Autodesk Inventor part; units mm, degrees
ref_plane "YZ Plane" through (0, 0, 0) normal (1, 0, 0) x (0, 1, 0)
ref_plane "XZ Plane" through (0, 0, 0) normal (0, 1, 0) x (-1, 0, 0)
ref_plane "XY Plane" through (0, 0, 0) normal (0, 0, 1) x (1, 0, 0)
sketch "Boceto1" plane through (0, 0, 0) normal (0, 1, 0) x (-1, 0, 0)
  line L0 (38.5, -14) -> (-38.5, -14)
  line L1 (-38.5, -14) -> (-38.5, 14)
  line L2 (-38.5, 14) -> (38.5, 14)
  line L3 (38.5, 14) -> (38.5, -14)
  circle A0 centre (-29.5, 6) radius 2.5
  circle A1 centre (-29.5, -6) radius 2.5
  point P0 (0, 0)
  point P1 (0, -14)
  point P2 (-38.5, 0)
  dimension "d0" = 5
  dimension "d1" = 9
  dimension "d2" = 77
  dimension "d3" = 28
  dimension "d17" = 8
  dimension "d18" = 5
  dimension "d19" = 12
extrude "Extrusión1" add sketch "Boceto1" along normal blind 9
sketch "Boceto2" plane through (0, 0, 0) normal (0, -1, 0) x (1, 0, 0)
  line L0 (-38.5, 14) -> (38.5, 14)
  line L1 (26.5, 14) -> (32.5, 14)
  line L2 (32.5, 14) -> (32.5, -14)
  line L3 (32.5, -14) -> (26.5, -14)
  line L4 (26.5, -14) -> (26.5, 14)
  line L5 (38.5, -14) -> (-38.5, -14)
  circle A0 centre (29.5, 6) radius 2.5
  circle A1 centre (29.5, -6) radius 2.5
  point P0 (0, 0)
  point P1 (29.5, 14)
  point P2 (26, 6)
  point P3 (31, 6)
  point P4 (26, -6)
  point P5 (31, -6)
  dimension "d6" = 6
extrude "Extrusión2" add sketch "Boceto2" along normal blind 1 contours L0 L2 L3 L4 | A0 | A1
sketch "Boceto3" plane through (0, 9, 0) normal (0, 1, 0) x (1, 0, 0)
  line L0 (-38.5, 14) -> (-38.5, -14)
  circle A0 centre (29.5, 6) radius 2.5
  circle A1 centre (29.5, -6) radius 2.5
  line L1 (38.5, -14) -> (38.5, 14)
  line L2 (38.5, 14) -> (-38.5, 14)
  line L3 (-38.5, -14) -> (38.5, -14)
  point P0 (0, 0)
  point P1 (-33.5, 6)
  point P2 (-33.5, -6)
  point P3 (15.5, -6)
  point P4 (15.5, 6)
  dimension "d9" = 5
  dimension "d25" = 14
hole "Agujero1" at (-33.5, 9, -6) at (-33.5, 9, 6) at (15.5, 9, 6) at (15.5, 9, -6) direction (0, -1, 0) diameter 4.5 end through all countersink diameter 8 countersink angle 90
sketch "Boceto4" plane through (0, 9, 0) normal (0, 1, 0) x (1, 0, 0)
  circle A0 centre (29.5, 6) radius 2.5
  circle A1 centre (29.5, -6) radius 2.5
  point P0 (0, 0)
hole "Agujero2" at (29.5, 9, -6) at (29.5, 9, 6) direction (0, -1, 0) diameter 4.134 depth 14.2 tip angle 118 countersink diameter 10 countersink angle 90
properties part number "Base sujecion centelladora"
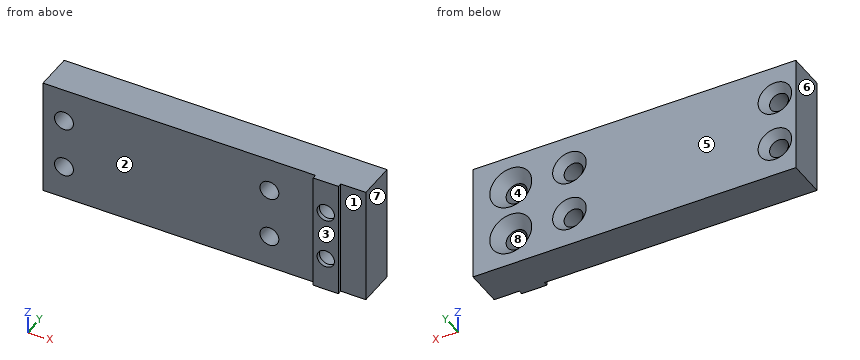
Model file for the job. Use its own axes, mm. Face numbers are marked on the shaded views. A direction names the side the tool comes from. Give positions to 0.01 mm unless a question says otherwise; leave off trailing zeros. Loops run counter-clockwise (first coordinate to the right, second up) from the corner with the lowest first, then second, coordinate; pieces in that order, holes last. Notation, with made-up numbers: (53.5, 41.5) -> (85.5, 41.5) arc R25 cw to (85.5, 56.5) -> close; hole circle Ø11 at (-22.75, -28). An arc over 180 degrees is marked (long way). Use CSV: the item, a comma, the result in double quotes. Start each with the question number.
1) Wall check: line 1 (X direction, y = 5, z = -6); line 2 (Z direction, x = 15.5, y = 1.5); line 3 (Z direction, x = 29.5, y = -0.35). Give the ranges that are in metal, low to high.
2) Slice it at C-C on y = 2.75. Give the cut face in (x, z).
3) Slice it at D-D on x = -33.5. Give the cut face in (y, z).
4) Mould opens along X. For the marked faces 6, 7 and 8 say: released by +X, released by -X, zero draft, split by the parting line, or undercut.
5) Slice it at A-A on x = 29.5. Give the cut face in (y, z).
6) Tool access for the marked faces 1, 2, 3, 4 and 5: list every direction of +Z, -Z, +X, -X, +Y, -Y with a clear straight run to the whole face (end or side of a thin tool).
7) Flat gauge pins, fed straight in: pin 1 Ø4 at (x, z) = (29.5, -5) entering from +Y; pin 2 Ø6 at (x, z) = (-33.5, -6) entering from +Y; pin 3 Ø0.8 at (y, z) = (-0.5, -1.5) entering from -X. Where does each tip first touch, or does it go through?
8) Slice it at B-B on z = -6. Give the number of separate pieces and of enclosed holes in the cut face, plus the area to 3 significant figures.
Computed values:
1,line 1,"x = -38.5 to -35.75, -31.25 to 13.25, 17.75 to 27, 32 to 38.5"
1,line 2,"z = -14 to -8.25, -3.75 to 3.75, 8.25 to 14"
1,line 3,"z = -14 to -8.07, -3.93 to 3.93, 8.07 to 14"
2,outline,"(-38.5, -14) -> (38.5, -14) -> (38.5, 14) -> (-38.5, 14) -> close; hole circle Ø4.5 at (-33.5, -6); hole circle Ø4.5 at (-33.5, 6); hole circle Ø4.5 at (15.5, -6); hole circle Ø4.5 at (15.5, 6); hole circle Ø5 at (29.5, -6); hole circle Ø5 at (29.5, 6)"
3,outline,"(0, -14) -> (9, -14) -> (9, -10) -> (7.25, -8.25) -> (0, -8.25) -> close; (0, -3.75) -> (7.25, -3.75) -> (9, -2) -> (9, 2) -> (7.25, 3.75) -> (0, 3.75) -> close; (0, 8.25) -> (7.25, 8.25) -> (9, 10) -> (9, 14) -> (0, 14) -> close"
4,face 6,"released by -X"
4,face 7,"released by +X"
4,face 8,"undercut"
5,outline,"(-1, -14) -> (9, -14) -> (9, -11) -> (6.5, -8.5) -> (0, -8.5) -> (0, -8.07) -> (-1, -8.07) -> close; (-1, -3.93) -> (0, -3.93) -> (0, -3.5) -> (6.5, -3.5) -> (9, -1) -> (9, 1) -> (6.5, 3.5) -> (0, 3.5) -> (0, 3.93) -> (-1, 3.93) -> close; (-1, 8.07) -> (0, 8.07) -> (0, 8.5) -> (6.5, 8.5) -> (9, 11) -> (9, 14) -> (-1, 14) -> close"
6,face 1,"+Z, -Z, +X, -Y"
6,face 2,"+Z, -Z, -X, -Y"
6,face 3,"+Z, -Z, +X, -X, -Y"
6,face 4,"+Y"
6,face 5,"+Z, -Z, +X, -X, +Y"
7,pin 1,"stops at y = 7"
7,pin 2,"stops at y = 8"
7,pin 3,"stops at x = 26.5"
8,separate pieces,"4"
8,enclosed holes,"0"
8,area,"556 mm^2"
